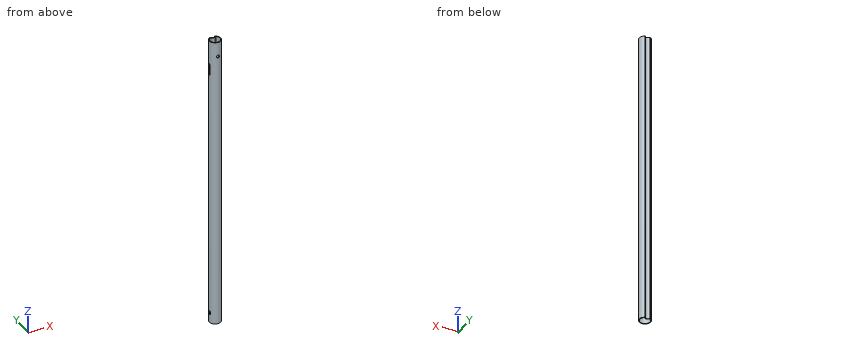
from build123d import *

# Parameters (mm, degrees)
ESTRUSIONE_ESTRUSIONE1_DEPTH = 200
SCHIZZO2_R                   = 1.5
TAGLIO_ESTRUSIONE1_DEPTH     = 200
SCHIZZO3_R                   = 1
TAGLIO_ESTRUSIONE2_DEPTH     = 200


with BuildPart() as part:
    # Schizzo1 → Estrusione-Estrusione1 (new body)
    with BuildSketch(Plane.XY):
        with BuildLine():
            ThreePointArc((-1.999681097, 3.464285714), (0, -4), (1.999681097, 3.464285714))
            ThreePointArc((1.999681097, 3.464285714), (1.615959904, 3.513025861), (1.31229072, 3.2734375))
            ThreePointArc((1.31229072, 3.2734375), (0, 2.5), (-1.31229072, 3.2734375))
            ThreePointArc((-1.31229072, 3.2734375), (-1.615959904, 3.513025861), (-1.999681097, 3.464285714))
        make_face()
        with BuildLine():
            ThreePointArc((-2.184763914, 2.734375), (0, -3.5), (2.184763914, 2.734375))
            ThreePointArc((2.184763914, 2.734375), (1.829579631, 2.841891076), (1.498123827, 2.675))
            ThreePointArc((1.498123827, 2.675), (0, 2), (-1.498123827, 2.675))
            ThreePointArc((-1.498123827, 2.675), (-1.829579631, 2.841891076), (-2.184763914, 2.734375))
        make_face(mode=Mode.SUBTRACT)
    extrude(amount=ESTRUSIONE_ESTRUSIONE1_DEPTH)

    # Schizzo2 → Taglio-Estrusione1 (cut)
    with BuildSketch(Plane(origin=(0, 0, 0), x_dir=(0, 0, -1), z_dir=(1, 0, 0))):
        with Locations((-7, 0)):
            Circle(SCHIZZO2_R)
        with BuildLine():
            Line((-183, 1), (-177, 1))
            ThreePointArc((-177, 1), (-176, 0), (-177, -1))
            Line((-177, -1), (-183, -1))
            ThreePointArc((-183, -1), (-184, 0), (-183, 1))
        make_face()
    extrude(amount=-TAGLIO_ESTRUSIONE1_DEPTH, mode=Mode.SUBTRACT)

    # Schizzo3 → Taglio-Estrusione2 (cut)
    with BuildSketch(Plane(origin=(0, 0, 0), x_dir=(1, 0, 0), z_dir=(0, 1, 0))):
        with Locations(Location((0, -190, 0), (0, 0, 270))):
            Circle(SCHIZZO3_R)
    extrude(amount=-TAGLIO_ESTRUSIONE2_DEPTH, mode=Mode.SUBTRACT)


solid = part.part
Geometry: final body of the model. Coordinates: model frame, mm. Round coordinates to 2 decimals unless told otherwise and drop trailing zeros. Loops run counter-clockwise (first coordinate to the right, second up) from the corner with the lowest first, then second, coordinate; pieces in that order, holes last. Notation, with made-up numbers: M -29.75,61.25 L -6.75,61.25 A27 ccw -6.75,98.25 Z; hole C -24,57 d4. An arc over 180 degrees is marked long. Put each result on its own line as item: value. Start each with the question number.
(1) Material intervals for line 1 along Z through (x, y) = (-3.55, 0); line 2 along X through (y, z) = (-0.5, 72.5); line 3 along X through (y, z) = (1.25, 24), sorted ascending. Write a range as [from, to].
(2) Contact query for flat-ended pins moving along their axis: pin 1 Ø1.5 at (x, z) = (2.5, 81) entering from -Y; pin 2 Ø1.2 at (x, z) = (0, 190) entering from +Y; pin 3 Ø1 at (y, z) = (-2.5, 76) entering from -X. Output: stop coordinate, or through.
(3) Section query A-A (z = 44). Return loops of the section in (x, y) (3 decimals), then the cut area to 3 significant figures.
Findings below:
1. line 1: z = [0, 5.5], [8.5, 176], [184, 200]
1. line 2: x = [-3.97, -3.46], [3.46, 3.97]
1. line 3: x = [-3.8, -3.27], [3.27, 3.8]
2. pin 1: stops at y = -3.6
2. pin 2: stops at y = 2.63
2. pin 3: stops at x = -3.46
3. outline: M -2,3.464 A4 ccw long 2,3.464 A0.5 ccw 1.312,3.273 A1.5 cw -1.312,3.273 A0.5 ccw Z; hole M -2.185,2.734 A3.5 ccw long 2.185,2.734 A0.5 ccw 1.498,2.675 A2 cw -1.498,2.675 A0.5 ccw Z
3. area: 12.2 mm2
